from build123d import *

# Parameters (mm, degrees)
SKETCH1_W           = 50
SKETCH1_H           = 25
BOSS_EXTRUDE1_DEPTH = 10
SKETCH2_R           = 1.5
CUT_EXTRUDE1_DEPTH  = 10
SKETCH3_R           = 1.4
CUT_EXTRUDE2_DEPTH  = 10
SKETCH4_R           = 2
CUT_EXTRUDE3_DEPTH  = 10
FILLET1_R           = 10
SKETCH5_R           = 3.5
CUT_EXTRUDE4_DEPTH  = 4


with BuildPart() as part:
    # Sketch1 → Boss-Extrude1 (new body)
    with BuildSketch(Plane(origin=(0, 0, 0), x_dir=(1, 0, 0), z_dir=(0, 1, 0))):
        Rectangle(SKETCH1_W, SKETCH1_H)
    extrude(amount=BOSS_EXTRUDE1_DEPTH)

    # Sketch2 → Cut-Extrude1 (cut)
    with BuildSketch(Plane(origin=(0, 10, 0), x_dir=(1, 0, 0), z_dir=(0, 1, 0))):
        with Locations(Location((-15, 5, 0), (0, 0, 270))):
            Circle(SKETCH2_R)
        with Locations(Location((-15, -5, 0), (0, 0, 270))):
            Circle(SKETCH2_R)
        with Locations(Location((15, -5, 0), (0, 0, 90))):
            Circle(SKETCH2_R)
        with Locations(Location((15, 5, 0), (0, 0, 90))):
            Circle(SKETCH2_R)
    extrude(amount=-CUT_EXTRUDE1_DEPTH, mode=Mode.SUBTRACT)

    # Sketch3 → Cut-Extrude2 (cut)
    with BuildSketch(Plane(origin=(0, 10, 0), x_dir=(1, 0, 0), z_dir=(0, 1, 0))):
        with Locations(Location((-6.717514421, -6.717514421, 0), (0, 0, 270))):
            Circle(SKETCH3_R)
        with Locations(Location((6.717514421, -6.717514421, 0), (0, 0, 270))):
            Circle(SKETCH3_R)
        with Locations(Location((6.717514421, 6.717514421, 0), (0, 0, 270))):
            Circle(SKETCH3_R)
        with Locations(Location((-6.717514421, 6.717514421, 0), (0, 0, 270))):
            Circle(SKETCH3_R)
    extrude(amount=-CUT_EXTRUDE2_DEPTH, mode=Mode.SUBTRACT)

    # Sketch4 → Cut-Extrude3 (cut)
    with BuildSketch(Plane(origin=(0, 10, 0), x_dir=(1, 0, 0), z_dir=(0, 1, 0))):
        with Locations(Location((0, 0, 0), (0, 0, 270))):
            Circle(SKETCH4_R)
    extrude(amount=-CUT_EXTRUDE3_DEPTH, mode=Mode.SUBTRACT)

    # Fillet1
    fillet1_edges = [part.edges().sort_by_distance(p)[0] for p in [
        (-25, 5, -12.5),
        (25, 5, -12.5),
        (25, 5, 12.5),
        (-25, 5, 12.5),
    ]]
    fillet(fillet1_edges, radius=FILLET1_R)

    # Sketch5 → Cut-Extrude4 (cut)
    with BuildSketch(Plane.XZ):
        with Locations(Location((-6.717514421, 6.717514421, 0), (0, 0, 270))):
            Circle(SKETCH5_R)
        with Locations(Location((6.717514421, 6.717514421, 0), (0, 0, 270))):
            Circle(SKETCH5_R)
        with Locations(Location((6.717514421, -6.717514421, 0), (0, 0, 270))):
            Circle(SKETCH5_R)
        with Locations(Location((-6.717514421, -6.717514421, 0), (0, 0, 270))):
            Circle(SKETCH5_R)
    extrude(amount=-CUT_EXTRUDE4_DEPTH, mode=Mode.SUBTRACT)


solid = part.part
Can you work these out from the model? Positions are in its coordinate system, mm. A direction names the side the tool comes from. Give positions to 0.01 mm unless a question says otherwise; leave off trailing zeros. Loops run counter-clockwise (first coordinate to the right, second up) from the corner with the lowest first, then second, coordinate; pieces in that order, holes last. Notation, with made-up numbers: M -19,1.25 L 16,1.25 A33 ccw 16,38.25 Z; hole C 9,77 d5. An arc over 180 degrees is marked long. One line per item, written item: value. Start each with the question number.
1) Thinking about a two-plate mould opening in Z: for faces 1 (the face through (-5.771, 7.042, 5.686)), 2 (the face through (0, 5, -12.5)), 3 (the face through (0, 10, -3)), which applies, +Z half, -Z half, draft (parallel to the pull), parting line (faces both ways), or undercut?
2) If we section it at B-B, the plane x = 0: Write out the boundary of the cut face in (y, z).
3) I'm going to push flat-ended pins straight in: pin 1 (1 mm diameter, centred on x = -4.5, z = 6.5, fed in from -Y); pin 2 (1.7 mm diameter, centred on x = 6.72, z = 6.72, fed in from +Y); pin 3 (5 mm diameter, centred on y = 6, z = -6.5, fed in from -X). Where does each tip first touch, or does it pass through?
4) If we section it at A-A, the plane z = -4.5: Write out the boundary of the cut face in (x, y).
5) If we section it at C-C, the plane z = 0: Write out the boundary of the cut face in (x, y), and give its area (3 significant figures).
6) On a 3-axis mill with a long thin cutter (end or side, diameter ignored), from which of +Z, -Z, +X, -X, +Y, -Y can I reach the whole of each face in a straight line? I mean faces 4 (the face through (-3.766, 1.972, 4.836)), 5 (the face through (14.93, 5.07, 6.5)). Say none if no direction works.
7) If we section it at D-D, the plane y = 6.75: Give the number of separate pieces and of enclosed holes in the cut face, and give its area (3 significant figures).
8) If I drill on line 1 (X direction, y = 2.5, z = -3.75); line 2 (X direction, y = 7, z = -5); line 3 (Z direction, x = 3.5, y = 3), over which ranges is the centre line in solid material (lowest first)? Write a range as [from, to].
Completed:
1. face 1: undercut
1. face 2: -Z half
1. face 3: draft
2. outline: M 0,-12.5 L 10,-12.5 L 10,-2 L 0,-2 Z; M 0,2 L 10,2 L 10,12.5 L 0,12.5 Z
3. pin 1: stops at y = 4
3. pin 2: passes through
3. pin 3: stops at x = -24.89
4. outline: M -24.8,0 L -16.41,0 L -16.41,10 L -24.8,10 Z; M -13.59,0 L -9.43,0 L -9.43,4 L -4.01,4 L -4.01,0 L 4.01,0 L 4.01,4 L 9.43,4 L 9.43,0 L 13.59,0 L 13.59,10 L -13.59,10 Z; M 16.41,0 L 24.8,0 L 24.8,10 L 16.41,10 Z
5. outline: M -25,0 L -2,0 L -2,10 L -25,10 Z; M 2,0 L 25,0 L 25,10 L 2,10 Z
5. area: 460 mm^2
6. face 4: -Y
6. face 5: +Y, -Y
7. separate pieces: 1
7. enclosed holes: 9
7. area: 1,100 mm^2
8. line 1: x = [-24.92, -15.83], [-14.17, -8.57], [-4.86, 4.86], [8.57, 14.17], [15.83, 24.92]
8. line 2: x = [-24.68, -16.5], [-13.5, 13.5], [16.5, 24.68]
8. line 3: z = [-12.5, -8.1], [-5.34, 5.34], [8.1, 12.5]
